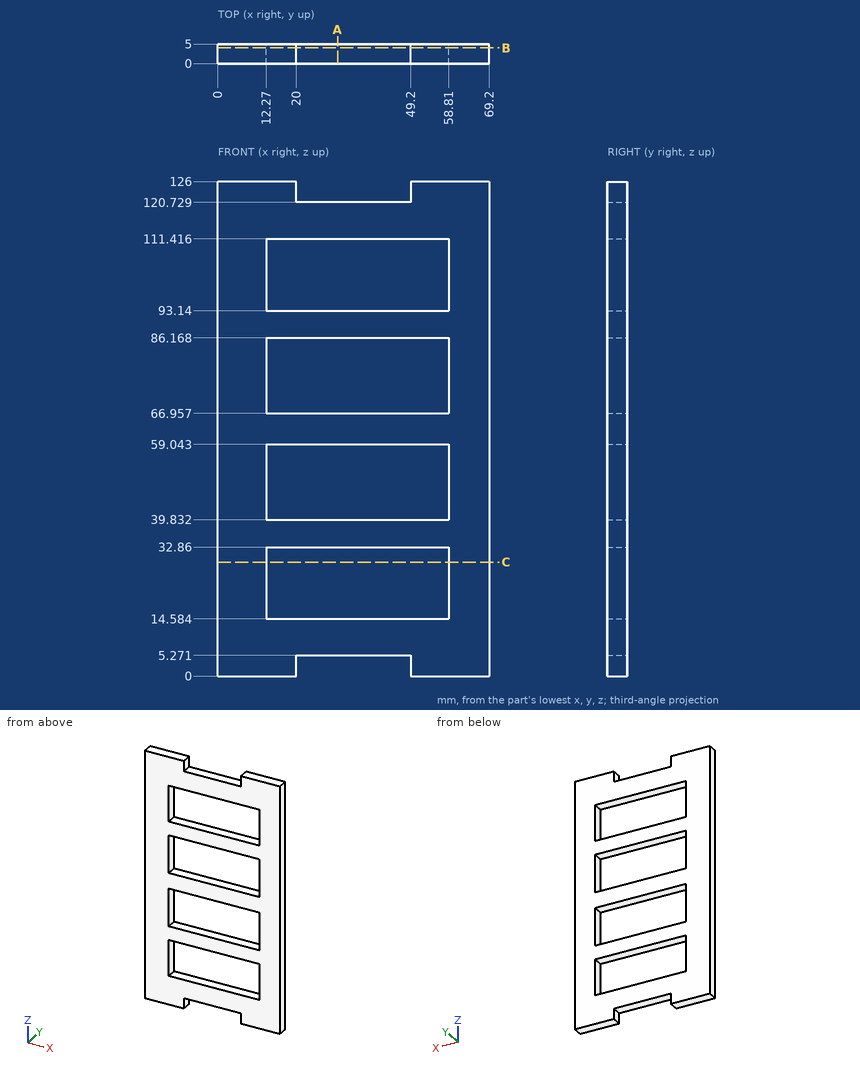
Could you check a few things on this drawing? It's one solid part, dimensions in mm from its lowest x, y, z. Give positions to 0.01 mm unless a question says otherwise; leave off trailing zeros. Write each loop counter-clockwise with the first axis right and the second up, starting at its lowest first coordinate (ties: lowest second). Pieces come first, ordered by that corner, then holes. Notation, with made-up numbers: (-12, 59.5) - (9, 59.5) arc R26 ccw to (9, 92.5) - close; hole circle Ø5 at (56.5, -1). An arc over 180 degrees is marked (long way). Use CSV: the item, a comma, the result in double quotes. Start each with the question number.
Item 1: I want a section at A-A, the plane x = 30.5. Please give me the cut outline in (y, z).
Item 2: I want a section at C-C, the plane z = 29. Please give me the cut outline in (x, y), then the cut area to 3 significant figures.
Item 3: I'm going to push flat-ended pins straight in: pin 1 (1.5 mm diameter, centred on x = 47, y = 2, fed in from +Z); pin 2 (2.5 mm diameter, centred on y = 2.5, z = 1.5, fed in from -X); pin 3 (1.5 mm diameter, centred on x = 40, y = 3.5, fed in from -Z). Where does each tip first touch, or does it pass through?
Item 4: I want a section at B-B, the plane y = 4. Please give me the cut outline in (x, z), then the cut area to 3 significant figures.
Item 5: If I drill on line 1 along Z through (x, y) = (15, 4.15); line 2 along Z through (x, y) = (37, 3.4); line 3 along X through (y, z) = (3.4, 24.5), over which ranges is the centre line in solid material (lowest first)?
Findings:
1,outline,"(0, 5.27) - (5, 5.27) - (5, 14.58) - (0, 14.58) - close; (0, 32.86) - (5, 32.86) - (5, 39.83) - (0, 39.83) - close; (0, 59.04) - (5, 59.04) - (5, 66.96) - (0, 66.96) - close; (0, 86.17) - (5, 86.17) - (5, 93.14) - (0, 93.14) - close; (0, 111.42) - (5, 111.42) - (5, 120.73) - (0, 120.73) - close"
2,outline,"(0, 0) - (12.27, 0) - (12.27, 5) - (0, 5) - close; (58.81, 0) - (69.2, 0) - (69.2, 5) - (58.81, 5) - close"
2,area,"113 mm2"
3,pin 1,"stops at z = 120.73"
3,pin 2,"stops at x = 0"
3,pin 3,"stops at z = 5.27"
4,outline,"(0, 0) - (20, 0) - (20, 5.27) - (49.2, 5.27) - (49.2, 0) - (69.2, 0) - (69.2, 126) - (49.2, 126) - (49.2, 120.73) - (20, 120.73) - (20, 126) - (0, 126) - close; hole (12.27, 14.58) - (58.81, 14.58) - (58.81, 32.86) - (12.27, 32.86) - close; hole (12.27, 39.83) - (58.81, 39.83) - (58.81, 59.04) - (12.27, 59.04) - close; hole (12.27, 66.96) - (58.81, 66.96) - (58.81, 86.17) - (12.27, 86.17) - close; hole (12.27, 93.14) - (58.81, 93.14) - (58.81, 111.42) - (12.27, 111.42) - close"
4,area,"4,920 mm2"
5,line 1,"z = 0 to 14.58, 32.86 to 39.83, 59.04 to 66.96, 86.17 to 93.14, 111.42 to 126"
5,line 2,"z = 5.27 to 14.58, 32.86 to 39.83, 59.04 to 66.96, 86.17 to 93.14, 111.42 to 120.73"
5,line 3,"x = 0 to 12.27, 58.81 to 69.2"
